Can you work these out from the model? Positions are in its coordinate system, mm. Face numbers are marked on the shaded views. A direction names the side the tool comes from. Coordinates: 2 decimals unless noted, no trailing zeros. Loops run counter-clockwise (first coordinate to the right, second up) from the corner with the lowest first, then second, coordinate; pieces in that order, holes last. Notation, with made-up numbers: M -39.75,-13 L 18.25,-13 A27 cw 18.25,15 Z; hole C -7,19.5 d5. An arc over 180 degrees is marked long. Answer as a JSON object with one key per item and string values. Group by question number.
Item 1: Suppose I cut it at A-A (z = 0.8). Write out the boundary of the cut face in (x, y).
Item 2: Suppose I cut it at B-B (y = -1.7). Write out the boundary of the cut face in (x, z).
Item 3: If I drill on line 1 (Y direction, x = 9.75, z = 1.4); line 2 (X direction, y = -0.2, z = 0.6); line 3 (X direction, y = 0.3, z = 1.4), over which ranges is the centre line in solid material (lowest first)?
Item 4: Which directions (+Z, -Z, +X, -X, +Y, -Y) give clear straight access to the entire face, cutting with the end or side of a thin tool? Please do the marked faces 4 and 5.
Item 5: Suppose I cut it at C-C (y = 1.6). Write out the boundary of the cut face in (x, z).
Item 6: We'd pull the mould along Y, two halves only. Please class the marked faces 1, 2 and 3: +Y half, -Y half, draft (parallel to the pull), parting line (faces both ways), or undercut.
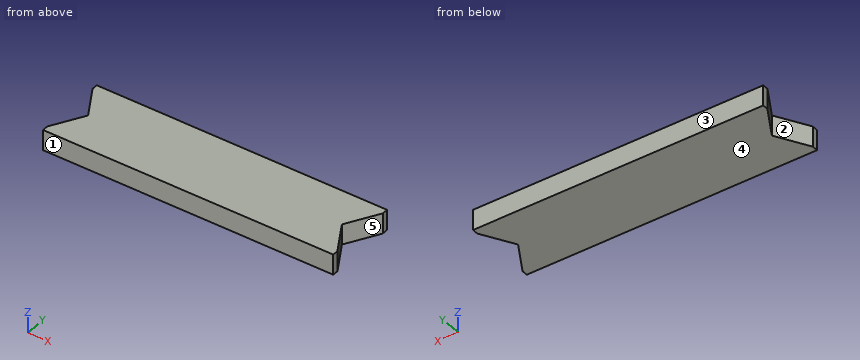
```python
from build123d import *

# Parameters (mm, degrees)
BOSS_EXTRUDE1_DEPTH = 1.5
SKETCH3_W           = 0.25
SKETCH3_H           = 5.5
CUT_EXTRUDE1_DEPTH  = 12.352995302


with BuildPart() as part:
    # Sketch2 → Boss-Extrude1 (new body)
    with BuildSketch(Plane.XY):
        Polygon((-10.91228676, 2.75), (-9.324573519, 0), (-10.91228676, -2.75), (10.91228676, -2.75), (9.324573519, 0), (10.91228676, 2.75), align=None)
    extrude(amount=BOSS_EXTRUDE1_DEPTH)

    # Sketch3 → Cut-Extrude1 (cut, through all)
    with BuildSketch(Plane.XY.offset(1.5)):
        with Locations((10.78728676, 0)):
            Rectangle(SKETCH3_W, SKETCH3_H)
        with Locations((-10.78728676, 0)):
            Rectangle(SKETCH3_W, SKETCH3_H)
    extrude(amount=-CUT_EXTRUDE1_DEPTH, mode=Mode.SUBTRACT)


solid = part.part
```
From the geometry:
{
 "1": {"outline": "M -10.66,-2.75 L 10.66,-2.75 L 10.66,-2.32 L 9.32,0 L 10.66,2.32 L 10.66,2.75 L -10.66,2.75 L -10.66,2.32 L -9.32,0 L -10.66,-2.32 Z"},
 "2": {"outline": "M -10.31,0 L 10.31,0 L 10.31,1.5 L -10.31,1.5 Z"},
 "3": {"line 1": "-2.75 to -0.74, 0.74 to 2.75", "line 2": "-9.44 to 9.44", "line 3": "-9.5 to 9.5"},
 "4": {"face 4": "-Z, +X, -X, +Y, -Y", "face 5": "+Z, -Z, +X"},
 "5": {"outline": "M -10.25,0 L 10.25,0 L 10.25,1.5 L -10.25,1.5 Z"},
 "6": {"face 1": "-Y half", "face 2": "undercut", "face 3": "+Y half"}
}
